Build history of the part. All positions in model axes, mm. A direction names the side the tool comes from. Round coordinates to 2 decimals unless told otherwise and drop trailing zeros. Loops run counter-clockwise (first coordinate to the right, second up) from the corner with the lowest first, then second, coordinate; pieces in that order, holes last. Notation, with made-up numbers: (47, 23.25) - (104, 23.25) arc R16 ccw to (104, 41.25) - close; hole circle Ø10 at (-15, 36.5). An arc over 180 degrees is marked (long way). Put each result on its own line as item: value. Start each with the question number.
from build123d import *

# Parameters (mm, degrees)
SKETCH1_W                    = 56
SKETCH1_H                    = 5
BOSS_EXTRUDE1_DEPTH          = 42
SKETCH2_W                    = 5
SKETCH2_H                    = 25
BOSS_EXTRUDE2_DEPTH          = 78
BOSS_EXTRUDE3_DEPTH          = 5
SKETCH5_W                    = 30
SKETCH5_H                    = 37
BOSS_EXTRUDE4_DEPTH          = 3
SKETCH9_W                    = 80
SKETCH9_H                    = 10
BOSS_EXTRUDE7_DEPTH          = 7.8
SKETCH6_R                    = 1.7
CUT_EXTRUDE1_DEPTH           = 10
SKETCH6_3_R                  = 1.7
CUT_EXTRUDE2_DEPTH           = 7.8
BOSS_EXTRUDE5_REACH          = 114.771
CUT_EXTRUDE3_START           = 3
CUT_EXTRUDE3_DEPTH           = 30
BOSS_EXTRUDE8_REACH          = 104.503
SKETCH12_W                   = 6
SKETCH12_H                   = 10
SKETCH14_W                   = 21.376587736
SKETCH14_H                   = 30
BOSS_EXTRUDE9_DEPTH          = 10
CUT_EXTRUDE4_DEPTH           = 113.771445038
SKETCH17_W                   = 20
SKETCH17_H                   = 15
CUT_EXTRUDE5_DEPTH           = 94.029704558
CUT_EXTRUDE6_DEPTH           = 126.411384609
BOSS_EXTRUDE11_DEPTH         = 70
CUT_EXTRUDE7_DEPTH           = 94.029704558
CUT_EXTRUDE8_DEPTH           = 97.630216889
BOSS_EXTRUDE12_DEPTH         = 1
M3_START                     = -53
M3_CLEARANCE_HOLE1_OUTLINE_R = 1.6
M3_CLEARANCE_HOLE1_DEPTH     = 12.039780493
BOSS_EXTRUDE13_REACH         = 111.463
SKETCH25_W                   = 15
SKETCH25_H                   = 40.960219507
BOSS_EXTRUDE14_DEPTH         = 12.039780493
SKETCH27_W                   = 18
SKETCH27_H                   = 11.5
BOSS_EXTRUDE15_DEPTH         = 5.614909
SKETCH28_R                   = 3
CUT_EXTRUDE9_DEPTH           = 38
CHAMFER4_SIZE                = 2
BOSS_EXTRUDE16_DEPTH         = 8.5
CUT_EXTRUDE10_DEPTH          = 108.068430529
BOSS_EXTRUDE17_DEPTH         = 37
CUT_EXTRUDE11_DEPTH          = 40
CUT_EXTRUDE11_DEPTH_BACK     = 137.170264842
SKETCH31_W                   = 22.2
SKETCH31_H                   = 27.6


# Read off the part's stored shape, not the designer's step: M3 Clearance Hole1
with BuildPart() as part:
    # Sketch1 → Boss-Extrude1 (new body)
    with BuildSketch(Plane(origin=(0, 0, 0), x_dir=(1, 0, 0), z_dir=(0, 1, 0))):
        with Locations((-2.5, -25.75)):
            Rectangle(SKETCH1_W, SKETCH1_H)
    extrude(amount=-BOSS_EXTRUDE1_DEPTH)

    # Sketch2 → Boss-Extrude2 (add)
    with BuildSketch(Plane(origin=(0, 0, 0), x_dir=(1, 0, 0), z_dir=(0, 1, 0))):
        with Locations((-28, -40.75)):
            Rectangle(SKETCH2_W, SKETCH2_H)
    extrude(amount=-BOSS_EXTRUDE2_DEPTH)

    # Sketch9 → Boss-Extrude7 (add)
    with BuildSketch(Plane(origin=(0, 0, 28.25), x_dir=(-1, 0, 0), z_dir=(0, 0, -1))):
        with Locations((-3.5, -47)):
            Rectangle(SKETCH9_W, SKETCH9_H)
    extrude(amount=BOSS_EXTRUDE7_DEPTH)


with BuildPart() as body_2:
    # Sketch4 → Boss-Extrude3 (new body)
    with BuildSketch(Plane(origin=(-51.961524227, 0, 30), x_dir=(-0.500000000000001, 0, -0.8660254037844382), z_dir=(0.866025403784438, 0, -0.5000000000000009))):
        Polygon((1.25, -53), (8.25, -43.002963953), (8.25, -37), (11.25, -37), (11.25, 0), (-13.75, 0), (-13.75, -53), align=None)
    extrude(amount=BOSS_EXTRUDE3_DEPTH)

    # Sketch6 → Cut-Extrude1 (cut)
    with BuildSketch(Plane(origin=(-51.961524227, 0, 30), x_dir=(0.5000000000000009, 0, 0.8660254037844383), z_dir=(-0.8660254037844382, 0, 0.5000000000000008))):
        Polygon((10, -11.5), (-4.5, -11.5), (-10, -18.054644759), (-10, -32.945355241), (-4.5, -39.5), (10, -39.5), align=None)
        with Locations((0, -5.5)):
            Circle(SKETCH6_R)
    extrude(amount=-CUT_EXTRUDE1_DEPTH, mode=Mode.SUBTRACT)

    # Sketch6<3> → Cut-Extrude2 (cut)
    with BuildSketch(Plane(origin=(-51.961524227, 0, 30), x_dir=(0.5000000000000009, 0, 0.8660254037844383), z_dir=(-0.8660254037844382, 0, 0.5000000000000008))):
        with Locations((0, -45.5)):
            Circle(SKETCH6_3_R)
    extrude(amount=-CUT_EXTRUDE2_DEPTH, mode=Mode.SUBTRACT)

    # Boss-Extrude5: up to this face of the body (flat: up to its plane)
    boss_extrude5_end = Plane(body_2.part.faces().sort_by_distance((-46.671460718, -53, 34.162658774))[0])
    # Sketch7 → Boss-Extrude5 (add, up to the picked face)
    with BuildSketch(Plane(origin=(0, 0, 0), x_dir=(1, 0, 0), z_dir=(0, 1, 0)), mode=Mode.PRIVATE) as boss_extrude5_sk1:
        Polygon((-45.086524227, -41.907849302), (-30.5, -41.907849302), (-30.5, -36.160254038), (-42.631397208, -36.160254038), (-40.756397208, -39.407849302), align=None)
    boss_extrude5_tool1 = split(extrude(boss_extrude5_sk1.sketch, amount=-BOSS_EXTRUDE5_REACH, mode=Mode.PRIVATE), bisect_by=boss_extrude5_end, keep=Keep.BOTH, mode=Mode.PRIVATE)

    add(part.part)  # Boss-Extrude5 merges part
    add(boss_extrude5_tool1.solids().sort_by(Axis((-36.415744, 0, 39.11699), (0, -1, 0)))[0])

    # Sketch11 → Cut-Extrude3 (cut)
    with BuildSketch(Plane(origin=(-47.631397208, 0, 27.5), x_dir=(-0.5000000000000007, 0, -0.8660254037844384), z_dir=(0.8660254037844383, 0, -0.5000000000000006)).offset(CUT_EXTRUDE3_START)):
        Polygon((4.5, -42), (4.5, -39.5), (10, -32.945355241), (10, -18.054644759), (4.5, -11.5), (-10.5, -11.5), (-10.5, -42), align=None)
    extrude(amount=CUT_EXTRUDE3_DEPTH, mode=Mode.SUBTRACT)

    # Sketch12 → Boss-Extrude8 (add, up to next)
    with BuildSketch(Plane.XY.offset(28.25), mode=Mode.PRIVATE) as boss_extrude8_sk1:
        with Locations((-33.5, -47)):
            Rectangle(SKETCH12_W, SKETCH12_H)
    boss_extrude8_tool1 = extrude(boss_extrude8_sk1.sketch, amount=BOSS_EXTRUDE8_REACH, mode=Mode.PRIVATE) - body_2.part
    add(boss_extrude8_tool1.solids().sort_by_distance((-33.5, -47, 28.25))[0])

    # Sketch14 → Boss-Extrude9 (add)
    with BuildSketch(Plane(origin=(12.865054877, -25.730109754, 22.282928689), x_dir=(0.8660254037844385, 0, -0.5000000000000004), z_dir=(0.3535533905932723, -0.7071067811865512, 0.6123724356957913))):
        with Locations((-39.001760389, -22.151235068)):
            Rectangle(SKETCH14_W, SKETCH14_H)
    extrude(amount=BOSS_EXTRUDE9_DEPTH)

    # Sketch15 → Cut-Extrude4 (cut, through all)
    with BuildSketch(Plane(origin=(0, 0, 0), x_dir=(1, 0, 0), z_dir=(0, 1, 0))):
        Polygon((-36.5, -36.160254038), (-36.5, -20.45), (-43.302739548, -24.377563509), align=None)
        Polygon((-36.5, -20.45), (-20.88676203, -20.45), (-24.790071522, -13.689269641), align=None)
        Polygon((-16.38342993, -28.25), (-25.5, -28.25), (-25.5, -46.759010276), (-10.647935899, -38.184167069), align=None)
        Polygon((-30.5, -41.907849302), (-33.181624327, -41.907849302), (-30.5, -46.552558883), align=None)
    extrude(amount=-CUT_EXTRUDE4_DEPTH, mode=Mode.SUBTRACT)

    # Sketch17 → Cut-Extrude5 (cut, through all)
    with BuildSketch(Plane(origin=(12.865054877, -25.730109754, 22.282928689), x_dir=(0.8660254037844385, 0, -0.5000000000000004), z_dir=(0.3535533905932723, -0.7071067811865512, 0.6123724356957913))):
        with Locations((-38.313466521, -30.509099445)):
            Rectangle(SKETCH17_W, SKETCH17_H)
    extrude(amount=-CUT_EXTRUDE5_DEPTH, mode=Mode.SUBTRACT)

    # Sketch18 → Cut-Extrude6 (cut, through all)
    with BuildSketch(Plane.ZY.offset(20.88676203)):
        Polygon((20.45, -42), (22.349523679, -42), (20.45, -44.193381015), align=None)
    extrude(amount=-CUT_EXTRUDE6_DEPTH, mode=Mode.SUBTRACT)

    # Sketch20 → Boss-Extrude11 (add)
    with BuildSketch(Plane.ZY.offset(19.790071522)):
        Polygon((23.25, -40.960219507), (22.349523679, -42), (23.25, -42), align=None)
    extrude(amount=-BOSS_EXTRUDE11_DEPTH)

    # Sketch21 → Cut-Extrude7 (cut, through all)
    with BuildSketch(Plane(origin=(12.865054877, -25.730109754, 22.282928689), x_dir=(0.935414346693486, 0.2672612419124244, -0.23145502494313555), z_dir=(-0.35355339059327223, 0.7071067811865507, -0.6123724356957918))):
        Polygon((-34.354012493, 9.239410059), (-34.909798545, 10.600802291), (-37.243131878, 10.600802291), (-36.354012493, 8.422913478), align=None)
    extrude(amount=CUT_EXTRUDE7_DEPTH, mode=Mode.SUBTRACT)

    # Sketch22 → Cut-Extrude8 (cut, through all)
    with BuildSketch(Plane.XZ.offset(52)):
        Polygon((-30.5, 28.25), (-30.5, 36.160254038), (-36.565698604, 36.160254038), (-36.5, 20.45), (-16.5, 20.45), (-16.5, 28.25), align=None)
    extrude(amount=CUT_EXTRUDE8_DEPTH, mode=Mode.SUBTRACT)

    # Sketch24 → Boss-Extrude12 (add)
    with BuildSketch(Plane.XZ.offset(52)):
        Polygon((-30.5, 36.160254038), (-36.5, 36.160254038), (-36.5, 20.45), (43.5, 20.45), (43.5, 28.25), (-25.5, 28.25), (-30.5, 28.25), align=None)
    extrude(amount=BOSS_EXTRUDE12_DEPTH)

    # M3 Clearance Hole1 outline → M3 Clearance Hole1 (cut)
    with BuildSketch(Plane(origin=(0, 0, 0), x_dir=(1, 0, 0), z_dir=(0, 1, 0)).offset(M3_START)):
        with Locations((-32.25, -24.25)):
            Circle(M3_CLEARANCE_HOLE1_OUTLINE_R)
        with Locations((32.25, -24.25)):
            Circle(M3_CLEARANCE_HOLE1_OUTLINE_R)
    extrude(amount=M3_CLEARANCE_HOLE1_DEPTH, mode=Mode.SUBTRACT)

    # Boss-Extrude13: up to this face of the body (flat: up to its plane)
    boss_extrude13_end = Plane(body_2.part.faces().sort_by_distance((-37.124420642, -23.2412407, 36.160254038))[0])
    # Sketch25 → Boss-Extrude13 (add, up to the picked face)
    with BuildSketch(Plane(origin=(5.25, 0, 9.09326674), x_dir=(-0.8660254037844383, 0, 0.5000000000000008), z_dir=(-0.5000000000000007, 0, -0.8660254037844382)), mode=Mode.PRIVATE) as boss_extrude13_sk1:
        with Locations((48.780544247, -20.480109754)):
            Rectangle(SKETCH25_W, SKETCH25_H)
    boss_extrude13_tool1 = split(extrude(boss_extrude13_sk1.sketch, amount=-BOSS_EXTRUDE13_REACH, mode=Mode.PRIVATE), bisect_by=boss_extrude13_end, keep=Keep.BOTH, mode=Mode.PRIVATE)
    add(boss_extrude13_tool1.solids().sort_by(Axis((-36.995191, -20.48011, 33.483539), (0.5000000000000007, 0, 0.8660254037844382)))[0])

    # Sketch26 → Boss-Extrude14 (add)
    with BuildSketch(Plane.XZ.offset(40.960219507)):
        Polygon((-36.5, 33.197640478), (-36.5, 36.160254038), (-41.631397208, 36.160254038), align=None)
    extrude(amount=BOSS_EXTRUDE14_DEPTH)

    # Sketch27 → Boss-Extrude15 (add)
    with BuildSketch(Plane(origin=(5.25, 0, 9.09326674), x_dir=(-0.8660254037844383, 0, 0.5000000000000008), z_dir=(-0.5000000000000007, 0, -0.8660254037844382))):
        with Locations((47.038774815, -5.75)):
            Rectangle(SKETCH27_W, SKETCH27_H)
    extrude(amount=BOSS_EXTRUDE15_DEPTH)

    # Sketch28 → Cut-Extrude9 (cut)
    with BuildSketch(Plane.XZ.offset(11.5)):
        with Locations((-32.25, 24.25)):
            Circle(SKETCH28_R)
    extrude(amount=CUT_EXTRUDE9_DEPTH, mode=Mode.SUBTRACT)

    # Chamfer4
    chamfer4_edges = [body_2.edges().sort_by_distance(p)[0] for p in [
        (3.5, -53, 20.45),
    ]]
    chamfer(chamfer4_edges, length=CHAMFER4_SIZE)

    # Sketch29 → Boss-Extrude16 (add)
    with BuildSketch(Plane(origin=(0, 0, 0), x_dir=(1, 0, 0), z_dir=(0, 1, 0))):
        Polygon((25.5, -23.25), (30.5, -23.25), (47.353915399, -32.980612592), (57.296460718, -15.759618943), (61.626587737, -18.259618943), (46.626587737, -44.240381057), (25.9, -44.240381057), (25.9, -28.25), (25.5, -28.25), align=None)
    extrude(amount=-BOSS_EXTRUDE16_DEPTH)

    # Sketch30<2> → Boss-Extrude17 (add)
    with BuildSketch(Plane.XZ.offset(8.5)):
        Polygon((46.626587737, 44.240381057), (44.028511525, 42.740381057), (59.028511525, 16.759618943), (61.626587737, 18.259618943), align=None)
    extrude(amount=BOSS_EXTRUDE17_DEPTH)

    # Sketch31 → Cut-Extrude11 (cut, two sides: drawn at the far end of the back side and taken through both)
    with BuildSketch(Plane(origin=(51.528511525, 0, 29.75), x_dir=(-0.5000000000000012, 0, 0.866025403784438), z_dir=(-0.8660254037844379, 0, -0.5000000000000011)).offset(-CUT_EXTRUDE11_DEPTH_BACK)):
        with Locations((0, -25.5)):
            Rectangle(SKETCH31_W, SKETCH31_H)
    extrude(amount=CUT_EXTRUDE11_DEPTH + CUT_EXTRUDE11_DEPTH_BACK, mode=Mode.SUBTRACT)


with BuildPart() as body_3:
    # Sketch5 → Boss-Extrude4 (new body)
    with BuildSketch(Plane(origin=(54.126587737, 0, 31.25), x_dir=(0.5000000000000011, 0, -0.866025403784438), z_dir=(0.866025403784438, 0, 0.5000000000000011))):
        with Locations((0, -27)):
            Rectangle(SKETCH5_W, SKETCH5_H)
    extrude(amount=-BOSS_EXTRUDE4_DEPTH)

    # Sketch30 → Cut-Extrude10 (cut, through all)
    with BuildSketch(Plane.XZ.offset(8.5)):
        Polygon((46.626587737, 44.240381057), (44.028511525, 42.740381057), (59.028511525, 16.759618943), (61.626587737, 18.259618943), align=None)
    extrude(amount=CUT_EXTRUDE10_DEPTH, mode=Mode.SUBTRACT)


solid = body_2.part
Item 1: Drop flat-ended pins along their axis: pin 1 Ø9 at (x, z) = (56.5, 33) entering from -Y; pin 2 Ø3 at (y, z) = (-47.5, 34) entering from -X; pin 3 Ø12 at (y, z) = (-14, 38.5) entering from +X. Give the stop position or say it passes through.
Item 2: Slice it at A-A (x = 28). Give the cut face in (y, z), plus the area to 3 significant figures.
Item 3: Slice it at D-D (z = 51.5). Give the cut face in (x, y).
Item 4: Slice it at C-C (x = -2). Give the cut face in (y, z).
Item 5: Drill centre lines: probe 1 along Z at (x, y) = (-32.25, -50.7); probe 2 along Z at (x, y) = (32, -46); probe 3 along X at (y, z) = (-50.8, 24.25). Where is each one in solid material? Low to high. Write a range as [from, to].
Item 6: Which spindle directions (+Z, -Z, +X, -X, +Y, -Y) get a long thin tool onto all of the face, cutting with end or side? Do faces 1 (the cylindrical face through (32.042, -47.064, 22.664)), 2 (the flat face through (58.4, -25.7, 20.9)), 3 (the flat face through (-28, -65, 28.25)). Say none if no direction does.
Item 7: Slice it at B-B (y = -25.5). Give the cut face in (x, z), plus the area to 3 significant figures.
Item 8: Two-plate mould, pull along X, no slides. Class faces 4 (the cylindrical face through (-33.43, -51.27, 23.17)), 5 (the flat face through (23, -11.7, 25)), 6 (the flat face through (54.23, -7.26, 31.07)): pulls with the +X half, pulls with the -X half, needs draft (parallel to the pull), parting line crosses it, or undercut.
Computed values:
1. pin 1: stops at y = -45.5
1. pin 2: stops at x = -50.52
1. pin 3: stops at x = 53.14
2. outline: (-53, 22.45) - (-51, 20.45) - (-44.19, 20.45) - (-40.96, 23.25) - (-42, 23.25) - (-42, 28.25) - (-53, 28.25) - close; (-8.5, 23.25) - (0, 23.25) - (0, 44.24) - (-8.5, 44.24) - close
2. area: 261 mm^2
3. outline: (-30.5, -78) - (-25.5, -78) - (-25.5, 0) - (-30.5, 0) - close
4. outline: (-53, 22.45) - (-51, 20.45) - (-44.19, 20.45) - (-40.96, 23.25) - (0, 23.25) - (0, 28.25) - (-53, 28.25) - close
5. probe 1: z = [20.45, 22.65], [25.85, 41.91]
5. probe 2: z = [20.45, 22.67], [25.83, 28.25]
5. probe 3: x = [-36.5, -33.85], [-30.65, 30.65], [33.85, 43.5]
6. face 1: -Y
6. face 2: +Z
6. face 3: -Z, +X, -X, -Y
7. outline: (-57.59, 20.26) - (-53.26, 17.76) - (-52.63, 18.84) - (-56.96, 21.34) - close; (-46.96, 38.66) - (-42.63, 36.16) - (-41.63, 36.16) - (-19.27, 23.25) - (18.07, 23.25) - (25.5, 27.54) - (25.5, 28.25) - (-25.5, 28.25) - (-25.5, 53.25) - (-30.5, 53.25) - (-30.5, 41.91) - (-45.09, 41.91) - close; (44.03, 42.74) - (45.98, 39.36) - (48.58, 40.86) - (46.63, 44.24) - close; (57.08, 20.14) - (59.03, 16.76) - (61.63, 18.26) - (59.68, 21.64) - close
7. area: 504 mm^2
8. face 4: undercut
8. face 5: needs draft
8. face 6: pulls with the +X half
